```python
from build123d import *

# Parameters (mm, degrees)
SKETCH004_W     = 44
SKETCH004_H     = 70.703306
PAD003_DEPTH    = 6
SKETCH006_W     = 5.5
SKETCH006_H     = 7
PAD004_DEPTH    = 50
PAD007_DEPTH    = 5
PAD008_DEPTH    = 5
SKETCH014_R     = 1.25
HOLE003_DEPTH   = 10
PAD010_DEPTH    = 7
POCKET_DEPTH    = 20
SKETCH017_W     = 38.3
SKETCH017_H     = 1.75
POCKET001_DEPTH = 60
CHAMFER003_SIZE = 1
PAD011_DEPTH    = 1


with BuildPart() as part:
    # Sketch004 → Pad003 (new body)
    with BuildSketch(Plane.XY.offset(-5)):
        with Locations((0, -19.648347)):
            Rectangle(SKETCH004_W, SKETCH004_H)
        with BuildLine():
            ThreePointArc((-13, -35), (0, -48), (13, -35))
            Line((13, -35), (13, 0))
            ThreePointArc((13, 0), (0, 13), (-13, 0))
            Line((-13, -35), (-13, 0))
        make_face(mode=Mode.SUBTRACT)
    extrude(amount=PAD003_DEPTH)

    # Sketch006 → Pad004 (join)
    with BuildSketch(Plane.XY):
        with Locations((-19.25, -51.5)):
            Rectangle(SKETCH006_W, SKETCH006_H)
        with Locations((19.25, -51.5)):
            Rectangle(SKETCH006_W, SKETCH006_H)
    extrude(amount=PAD004_DEPTH)

    # Sketch011 → Pad007 (join)
    with BuildSketch(Plane(origin=(17, 0, -4), x_dir=(0, 1, 0), z_dir=(1, 0, 0))):
        Polygon((-21.25, 5), (-48.25, 32), (-48.25, 28), (-25.25, 5), align=None)
    extrude(amount=PAD007_DEPTH)

    # Sketch012 → Pad008 (join)
    with BuildSketch(Plane(origin=(-17, 0, -4), x_dir=(0, 1, 0), z_dir=(1, 0, 0))):
        Polygon((-48.25, 32), (-48.25, 28), (-25.25, 5), (-21.25, 5), align=None)
    extrude(amount=-PAD008_DEPTH)

    # Sketch014 → Hole003 (cut)
    with BuildSketch(Plane.XY.offset(-5)):
        with Locations((-11.5, -51)):
            Circle(SKETCH014_R)
        with Locations((11.5, -51)):
            Circle(SKETCH014_R)
    extrude(amount=HOLE003_DEPTH, mode=Mode.SUBTRACT)

    # Sketch016 → Pad010 (join)
    with BuildSketch(Plane.XY.offset(1)):
        with BuildLine():
            ThreePointArc((-13, 11), (-17.5, 15.5), (-22, 11))
            Line((-22, 11), (-22, -10))
            ThreePointArc((-22, -10), (-17.5, -14.5), (-13, -10))
            Line((-13, 11), (-13, -10))
        make_face()
        with BuildLine():
            ThreePointArc((22, 11), (17.5, 15.5), (13, 11))
            Line((13, 11), (13, -10))
            ThreePointArc((13, -10), (17.5, -14.5), (22, -10))
            Line((22, 11), (22, -10))
        make_face()
    extrude(amount=PAD010_DEPTH)

    # Sketch015 → Pocket (cut)
    with BuildSketch(Plane.XY.offset(-5)):
        with BuildLine():
            ThreePointArc((-15.8, 10.7), (-17.5, 12.4), (-19.2, 10.7))
            Line((-19.2, 10.7), (-19.2, -9.3))
            ThreePointArc((-19.2, -9.3), (-17.5, -11), (-15.8, -9.3))
            Line((-15.8, 10.7), (-15.8, -9.3))
        make_face()
        with BuildLine():
            ThreePointArc((19.2, 10.7), (17.5, 12.4), (15.8, 10.7))
            Line((15.8, 10.7), (15.8, -9.3))
            ThreePointArc((15.8, -9.3), (17.5, -11), (19.2, -9.3))
            Line((19.2, 10.7), (19.2, -9.3))
        make_face()
    extrude(amount=POCKET_DEPTH, mode=Mode.SUBTRACT)

    # Sketch017 → Pocket001 (cut)
    with BuildSketch(Plane.XY.offset(-2)):
        with Locations((0, -50.875)):
            Rectangle(SKETCH017_W, SKETCH017_H)
    extrude(amount=POCKET001_DEPTH, mode=Mode.SUBTRACT)

    # Chamfer003
    chamfer003_edges = [part.edges().sort_by_distance(p)[0] for p in [
        (-22, -55, 0.5),
        (-22, -55, 25.5),
        (22, -55, 0.5),
        (22, -55, 25.5),
        (-19.25, -55, 50),
        (-22, -51.5, 50),
        (-19.25, -48, 50),
        (19.25, -55, 50),
        (22, -51.5, 50),
        (19.25, -48, 50),
        (-19.15, -50.875, 50),
        (19.15, -50.875, 50),
        (0, -55, -5),
    ]]
    chamfer(chamfer003_edges, length=CHAMFER003_SIZE)

    # Sketch018 → Pad011 (join, symmetric)
    with BuildSketch(Plane.XZ.offset(54)):
        Polygon((-16.5, 0), (-16.5, 5), (-11.5, 0), align=None)
        Polygon((16.5, 0), (16.5, 5), (11.5, 0), align=None)
    extrude(amount=PAD011_DEPTH, both=True)


solid = part.part
```
Geometry check sheet. Reference: the model listing, model coordinates, mm. A direction names the side the tool comes from. Round coordinates to 2 decimals unless told otherwise and drop trailing zeros. Order: outer loops, then holes, each group sorted by start corner. A loop starts at its lowest first (then second) coordinate and runs counter-clockwise, first axis right, second up. Notation, with made-up numbers: (-21.5, 49) -> (-9.5, 49) arc R19 cw to (-9.5, 84) -> close; hole circle Ø3 at (-1.5, 79). An arc over 180 degrees is marked (long way). Return JSON: item names as keys, results as strings. Group by question number.
Q1. Tool access check on faces 4 (the cylindrical face through (0, 13, -2)), 5 (the flat face through (17, -36, 13)), 6 (the cylindrical face through (-17.4, 15.5, 4.5)), 7 (the flat face through (-19.46, -36.78, 12.53)). Record the directions out of +Z, -Z, +X, -X, +Y, -Y that give a thin tool (end or side, any length) a straight path to the whole face; none if there is none.
Q2. Gauge pin test, flat ends, axial feed: pin 1 (6 mm diameter, centred on x = 13, z = 21, fed in from -Y); pin 2 (4 mm diameter, centred on x = 15.5, z = 44, fed in from +Y); pin 3 (1.4 mm diameter, centred on x = -15.5, y = -51, fed in from +Z); pin 4 (3 mm diameter, centred on x = 11.5, y = -51, fed in from +Z). Record the tip position at first contact, or that the pin passes through.
Q3. Release check for a two-part mould opening along Z. For faces 1 (the flat face through (-16.5, -49, 25)), 2 (the flat face through (-15.6, 0.7, 8)), 3 (the flat face through (16.8, -48, 24.7)) record: released by +Z, released by -Z, zero draft, split by the parting line, or undercut.
Q4. Section check C-C, the plane y = -2. Record the boundary of the cut face in (x, z), plus the area to 3 significant figures.
Q5. Section check D-D, the plane x = -18. Record the boundary of the cut face in (y, z).
Q6. Section check A-A, the plane x = 0. Record the boundary of the cut face in (y, z), plus the area to 3 significant figures.
Q7. Material ranges on probe 1 along X at (y, z) = (-51, -3.6); probe 2 along X at (y, z) = (-51, -1.9); probe 3 along X at (y, z) = (-4.5, 1), recorded low to high. Write a range as from..to.
Q8. Section check B-B, the plane z = 0. Count the separate pieces of the cut face and the enclosed holes in it, plus the area to 3 significant figures.
Numbers:
{
 "1": {"face 4": "+Z, -Z", "face 5": "+Z", "face 6": "+Z, +Y", "face 7": "+X, -X"},
 "2": {"pin 1": "through", "pin 2": "y = -48", "pin 3": "z = -2", "pin 4": "z = 1"},
 "3": {"face 1": "zero draft", "face 2": "released by +Z", "face 3": "undercut"},
 "4": {"outline": "(-22, -5) -> (-19.2, -5) -> (-19.2, 8) -> (-22, 8) -> close; (-15.8, -5) -> (-13, -5) -> (-13, 8) -> (-15.8, 8) -> close; (13, -5) -> (15.8, -5) -> (15.8, 8) -> (13, 8) -> close; (19.2, -5) -> (22, -5) -> (22, 8) -> (19.2, 8) -> close", "area": "146 mm^2"},
 "5": {"outline": "(-55, -4) -> (-54, -5) -> (-10.92, -5) -> (-10.92, 8) -> (-14.47, 8) -> (-14.47, 1) -> (-21.25, 1) -> (-48, 27.75) -> (-48, 49) -> (-49, 50) -> (-50, 50) -> (-50, -2) -> (-51.75, -2) -> (-51.75, 50) -> (-54, 50) -> (-55, 49) -> close; (12.32, -5) -> (15.7, -5) -> (15.7, 1) -> (15.47, 1) -> (15.47, 8) -> (12.32, 8) -> close; hole (-48, 1) -> (-25.25, 1) -> (-48, 23.75) -> close"},
 "6": {"outline": "(-55, -4) -> (-54, -5) -> (-48, -5) -> (-48, 1) -> (-50, 1) -> (-50, -2) -> (-51.75, -2) -> (-51.75, 1) -> (-55, 1) -> close; (13, -5) -> (15.7, -5) -> (15.7, 1) -> (13, 1) -> close", "area": "52.5 mm^2"},
 "7": {"probe 1": "-22..-12.75, -10.25..10.25, 12.75..22", "probe 2": "-22..-19.15, 19.15..22", "probe 3": "-22..-19.2, -15.8..-13, 13..15.8, 19.2..22"},
 "8": {"separate pieces": "1", "enclosed holes": "4", "area": "1,450 mm^2"}
}
